Geometry: final body of the model. Coordinates: model frame, mm. Coordinates: 2 decimals unless noted, no trailing zeros. Write each loop counter-clockwise with the first axis right and the second up, starting at its lowest first coordinate (ties: lowest second). Pieces come first, ordered by that corner, then holes. Notation, with made-up numbers: (30.25, 46) - (62.25, 46) arc R27 ccw to (62.25, 65) - close; hole circle Ø7 at (-9.5, -9.5). An arc over 180 degrees is marked (long way). Put each result on its own line as item: value.
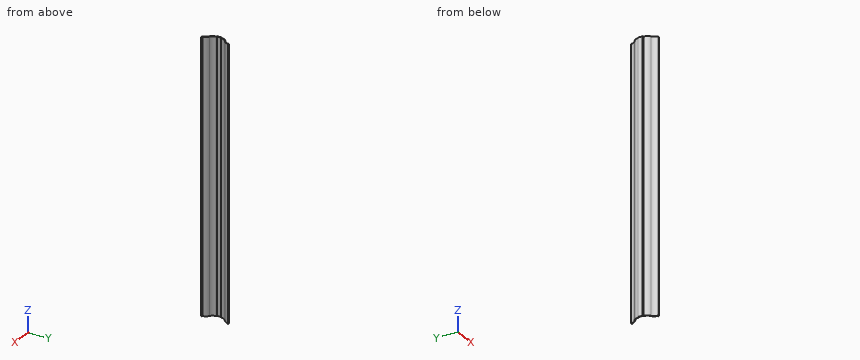
```python
from build123d import *

# Parameters (mm, degrees)
EXTRUDE_THIN1_DEPTH = 476.25
FILLET1_R           = 1.016


with BuildPart() as part:
    # Sketch1 → Extrude-Thin1 (new body)
    with BuildSketch(Plane.XY):
        with BuildLine():
            Line((0, 0), (-2.38125, 0))
            ThreePointArc((-2.38125, 0), (-3.753941176, 5.416289675), (-7.540625, 9.525))
            ThreePointArc((-7.540625, 9.525), (-11.327308824, 13.633710325), (-12.7, 19.05))
            Line((-12.7, 19.05), (-14.2875, 19.05))
            Line((-14.2875, 19.05), (-14.2875, 28.575))
            Line((-14.2875, 28.575), (-12.7, 28.575))
            ThreePointArc((-12.7, 28.575), (-11.327308824, 33.991289675), (-7.540625, 38.1))
            ThreePointArc((-7.540625, 38.1), (-3.753941176, 42.208710325), (-2.38125, 47.625))
            Line((-2.38125, 47.625), (0, 47.625))
            Line((0, 47.625), (0, 46.609))
            Line((0, 46.609), (-1.40698386, 46.609))
            ThreePointArc((-1.40698386, 46.609), (-3.111914342, 41.282721024), (-6.985575336, 37.249014765))
            ThreePointArc((-6.985575336, 37.249014765), (-10.665203574, 33.054213727), (-11.634040924, 27.559))
            Line((-11.634040924, 27.559), (-13.2715, 27.559))
            Line((-13.2715, 27.559), (-13.2715, 20.066))
            Line((-13.2715, 20.066), (-11.634040924, 20.066))
            ThreePointArc((-11.634040924, 20.066), (-10.665203574, 14.570786273), (-6.985575336, 10.375985235))
            ThreePointArc((-6.985575336, 10.375985235), (-3.111914342, 6.342278976), (-1.40698386, 1.016))
            Line((-1.40698386, 1.016), (0, 1.016))
            Line((0, 1.016), (0, 0))
        make_face()
    extrude(amount=-EXTRUDE_THIN1_DEPTH)

    # Fillet1
    fillet1_edges = [part.edges().sort_by_distance(p)[0] for p in [
        (-2.38125, 0, -238.125),
        (-14.2875, 19.05, -238.125),
        (-14.2875, 28.575, -238.125),
        (-2.38125, 47.625, -238.125),
        (-11.634040924, 27.559, -238.125),
        (-11.634040924, 20.066, -238.125),
    ]]
    fillet(fillet1_edges, radius=FILLET1_R)


solid = part.part
```
1. Pin query (flat end, axial travel): pin 1 Ø0.5 at (x, z) = (-13, -170.5) entering from -Y; pin 2 Ø5 at (x, z) = (-7, -255.5) entering from +Y; pin 3 Ø6 at (x, z) = (-6.5, -351) entering from -Y. Return the tip coordinate at first contact, or that it passes through.
Answer below:
pin 1: stops at y = 19.05
pin 2: stops at y = 41.01
pin 3: stops at y = 4.92
2. Section query B-B (y = 42). Return loops of the section in (x, z), then the cut area to 3 significant figures.
Answer below:
outline: (-3.87, -476.25) - (-2.72, -476.25) - (-2.72, 0) - (-3.87, 0) - close
area: 550 mm²
3. Ray query, probe 1 along Y at (x, z) = (-1, -79) (3 decimals); probe 2 along X at (y, z) = (20.5, -300.5); probe 3 along Y at (x, z) = (-13.5, -107.5). Return the intervals inside material, ascending. Write a range as from..to.
Answer below:
probe 1: y = 0..1.016, 46.609..47.625
probe 2: x = -14.29..-13.27
probe 3: y = 19.08..28.55
